Autodesk Inventor part; units mm, degrees
ref_plane "Work Plane1" through (72.9281, -13.9152, 0) normal (1, 0, 0) x (0, 0, -1)
ref_plane "YZ Plane" through (0, 0, 0) normal (1, 0, 0) x (0, 1, 0)
ref_plane "XZ Plane" through (0, 0, 0) normal (0, 1, 0) x (-1, 0, 0)
sketch "Sketch1" plane through (0, 0, 0) normal (0, 0, 1) x (1, 0, 0)
  line L0 (-25.0719, 9.0848) -> (170.9281, 9.0848)
  line L1 (172.9281, 7.0848) -> (172.9281, -13.9152)
  line L2 (170.9281, -15.9152) -> (-25.0719, -15.9152)
  line L3 (-27.0719, -13.9152) -> (-27.0719, 7.0848)
  arc A0 (-25.0719, 9.0848) -> (-27.0719, 7.0848) centre (-25.0719, 7.0848) ccw
  arc A1 (-27.0719, -13.9152) -> (-25.0719, -15.9152) centre (-25.0719, -13.9152) ccw
  arc A2 (170.9281, -15.9152) -> (172.9281, -13.9152) centre (170.9281, -13.9152) ccw
  arc A3 (172.9281, 7.0848) -> (170.9281, 9.0848) centre (170.9281, 7.0848) ccw
  point P0 (0, 0)
  point P1 (172.9281, -15.9152)
  point P2 (172.9281, 9.0848)
  point P3 (-27.0719, -15.9152)
  dimension "d0" = 200
  dimension "d1" = 25
  dimension "d2" = 2
extrude "Extrusion1" add sketch "Sketch1" along normal blind 2
sketch "Sketch2" plane through (0, 0, 2) normal (0, 0, 1) x (1, 0, 0)
  line L0 (170.9281, -15.9152) -> (-25.0719, -15.9152)
  line L1 (72.9281, -15.9152) -> (72.9281, 9.0848)
  line L2 (170.9281, 9.0848) -> (-25.0719, 9.0848)
  line L3 (-27.0719, 7.0848) -> (-27.0719, -13.9152)
  line L4 (-27.0719, -3.4152) -> (172.9281, -3.4152)
  line L5 (172.9281, 7.0848) -> (172.9281, -13.9152)
  circle A0 centre (-12.0719, -3.4152) radius 7.5
  line L6 (7.9281, -3.4152) -> (27.9281, -3.4152) construction
  line L7 (12.9281, -8.4152) -> (22.9281, -8.4152)
  line L8 (22.9281, 1.5848) -> (12.9281, 1.5848)
  arc A1 (12.9281, 1.5848) -> (12.9281, -8.4152) centre (12.9281, -3.4152) ccw
  arc A2 (22.9281, -8.4152) -> (22.9281, 1.5848) centre (22.9281, -3.4152) ccw
  line L9 (37.9281, -3.4152) -> (57.9281, -3.4152) construction
  line L10 (42.9281, 1.5848) -> (52.9281, 1.5848)
  line L11 (52.9281, -8.4152) -> (42.9281, -8.4152)
  arc A3 (42.9281, 1.5848) -> (42.9281, -8.4152) centre (42.9281, -3.4152) ccw
  arc A4 (52.9281, -8.4152) -> (52.9281, 1.5848) centre (52.9281, -3.4152) ccw
  point P0 (0, 0)
  point P1 (17.9281, -3.4152)
  point P2 (47.9281, -3.4152)
  dimension "d5" = 15
  dimension "d6" = 15
  dimension "d7" = 20
  dimension "d8" = 10
  dimension "d9" = 20
  dimension "d10" = 30
  dimension "d11" = 25
extrude "Extrusion2" cut sketch "Sketch2" against normal blind 2
ref_plane "Work Plane1" through (72.9281, -13.9152, 0) normal (1, 0, 0) x (0, 0, -1)
mirror "Mirror1" about plane through (72.9281, -13.9152, 0) normal (1, 0, 0) of "Extrusion2"
properties part number "Side Plate"
Verification items for the finished model (mm, model axes). A direction names the side the tool comes from. Give positions to 0.01 mm unless a question says otherwise; leave off trailing zeros. Loops run counter-clockwise (first coordinate to the right, second up) from the corner with the lowest first, then second, coordinate; pieces in that order, holes last.
1. Section check C-C, the plane z = 0.7. Enter the section's corners in (x, y).
2. Set-up check for faces 3 (the flat face through (72, -3, 2)), 4 (the cylindrical face through (57.927, -3.525, 1.014)): record each of +Z, -Z, +X, -X, +Y, -Y from which the full face is reachable in a straight line by a thin tool's end or side.
3. Go/stop test with flat-tipped pins: pin 1 Ø10 at (x, y) = (48.5, 2) entering from -Z; pin 2 Ø12 at (x, y) = (-12.07, -3.42) entering from +Z. Record where each tip stops, or that it passes through.
4. Section check A-A, the plane x = 48.5. Enter the section's corners in (y, z).
5. Mould release check, pull along X, two halves, no side actions. Record for faces 1 (the flat face through (72, -3, 0)), 2 (the cylindrical face through (117.93, -3.31, 1.01)): released by +X, released by -X, zero draft, split by the parting line, or undercut.
6. Thickness scan on line 1 (X direction, y = -10, z = 1.2); line 2 (Y direction, x = 95, z = 0.2); line 3 (X direction, y = 7.25, z = 1.15). Record the ranges inside material, lowest first.
7. Section check B-B, the plane y = -6.25. Enter the section's corners in (x, z).
8. Section check D-D, the plane x = -9. Enter the section's corners in (y, z), then the cut area to 3 significant figures.
Geometry says:
1. outline: (-27.07, -13.92) arc R2 ccw to (-25.07, -15.92) - (170.93, -15.92) arc R2 ccw to (172.93, -13.92) - (172.93, 7.08) arc R2 ccw to (170.93, 9.08) - (-25.07, 9.08) arc R2 ccw to (-27.07, 7.08) - close; hole circle Ø15 at (-12.07, -3.42); hole (12.93, -8.42) - (22.93, -8.42) arc R5 ccw to (22.93, 1.58) - (12.93, 1.58) arc R5 ccw to start; hole (42.93, -8.42) - (52.93, -8.42) arc R5 ccw to (52.93, 1.58) - (42.93, 1.58) arc R5 ccw to start; hole (92.93, -8.42) - (102.93, -8.42) arc R5 ccw to (102.93, 1.58) - (92.93, 1.58) arc R5 ccw to start; hole (122.93, -8.42) - (132.93, -8.42) arc R5 ccw to (132.93, 1.58) - (122.93, 1.58) arc R5 ccw to start; hole circle Ø15 at (157.93, -3.42)
2. face 3: +Z, +X, -X, +Y, -Y
2. face 4: +Z, -Z
3. pin 1: stops at z = 0
3. pin 2: passes through
4. outline: (-15.92, 0) - (-8.42, 0) - (-8.42, 2) - (-15.92, 2) - close; (1.58, 0) - (9.08, 0) - (9.08, 2) - (1.58, 2) - close
5. face 1: zero draft
5. face 2: undercut
6. line 1: x = -27.07 to -15.66, -8.48 to 154.34, 161.52 to 172.93
6. line 2: y = -15.92 to -8.42, 1.58 to 9.08
6. line 3: x = -27.07 to 172.92
7. outline: (-27.07, 0) - (-19.02, 0) - (-19.02, 2) - (-27.07, 2) - close; (-5.13, 0) - (8.81, 0) - (8.81, 2) - (-5.13, 2) - close; (27.05, 0) - (38.81, 0) - (38.81, 2) - (27.05, 2) - close; (57.05, 0) - (88.81, 0) - (88.81, 2) - (57.05, 2) - close; (107.05, 0) - (118.81, 0) - (118.81, 2) - (107.05, 2) - close; (137.05, 0) - (150.98, 0) - (150.98, 2) - (137.05, 2) - close; (164.87, 0) - (172.93, 0) - (172.93, 2) - (164.87, 2) - close
8. outline: (-15.92, 0) - (-10.26, 0) - (-10.26, 2) - (-15.92, 2) - close; (3.43, 0) - (9.08, 0) - (9.08, 2) - (3.43, 2) - close
8. area: 22.6 mm2
